from build123d import *

# Parameters (mm, degrees)
SKETCH_1_W      = 450
SKETCH_1_H      = 400
EXTRUDE_1_DEPTH = 50
SKETCH_2_W      = 50
SKETCH_2_H      = 50
EXTRUDE_2_DEPTH = 450
SKETCH_3_W      = 50
SKETCH_3_H      = 50
EXTRUDE_3_DEPTH = 450
SKETCH_4_W      = 50
SKETCH_4_H      = 50
EXTRUDE_4_DEPTH = 450
SKETCH_5_W      = 50
SKETCH_5_H      = 50
EXTRUDE_5_DEPTH = 450
SKETCH_6_W      = 400
SKETCH_6_H      = 80
EXTRUDE_6_DEPTH = 400
SKETCH_7_W      = 80
SKETCH_7_H      = 350
EXTRUDE_7_DEPTH = 250
SKETCH_8_W      = 80
SKETCH_8_H      = 350
EXTRUDE_8_DEPTH = 250


with BuildPart() as part:
    # 草图1 → 凸台-拉伸1 (new body)
    with BuildSketch(Plane.XY):
        Rectangle(SKETCH_1_W, SKETCH_1_H)
    extrude(amount=EXTRUDE_1_DEPTH)

    # 草图2 → 凸台-拉伸2 (add)
    with BuildSketch(Plane.XY):
        with Locations((-200, -175)):
            Rectangle(SKETCH_2_W, SKETCH_2_H)
    extrude(amount=EXTRUDE_2_DEPTH)

    # 草图3 → 凸台-拉伸3 (add)
    with BuildSketch(Plane.XY):
        with Locations((200, -175)):
            Rectangle(SKETCH_3_W, SKETCH_3_H)
    extrude(amount=EXTRUDE_3_DEPTH)

    # 草图4 → 凸台-拉伸4 (add)
    with BuildSketch(Plane.XY):
        with Locations((-200, 175)):
            Rectangle(SKETCH_4_W, SKETCH_4_H)
    extrude(amount=EXTRUDE_4_DEPTH)

    # 草图5 → 凸台-拉伸5 (add)
    with BuildSketch(Plane.XY):
        with Locations((200, 175)):
            Rectangle(SKETCH_5_W, SKETCH_5_H)
    extrude(amount=EXTRUDE_5_DEPTH)

    # 草图6 → 凸台-拉伸6 (add)
    with BuildSketch(Plane(origin=(0, 200, 0), x_dir=(1, 0, 0), z_dir=(0, 1, 0))):
        with Locations((0, -200)):
            Rectangle(SKETCH_6_W, SKETCH_6_H)
    extrude(amount=EXTRUDE_6_DEPTH)

    # 草图7 → 凸台-拉伸7 (add)
    with BuildSketch(Plane(origin=(0, 200, 0), x_dir=(1, 0, 0), z_dir=(0, 1, 0))):
        with Locations((-250, 0)):
            Rectangle(SKETCH_7_W, SKETCH_7_H)
    extrude(amount=EXTRUDE_7_DEPTH)

    # 草图8 → 凸台-拉伸8 (add)
    with BuildSketch(Plane(origin=(0, 200, 0), x_dir=(1, 0, 0), z_dir=(0, 1, 0))):
        with Locations((250, 0)):
            Rectangle(SKETCH_8_W, SKETCH_8_H)
    extrude(amount=EXTRUDE_8_DEPTH)


solid = part.part
Can you work these out from the model? Positions are in its coordinate system, mm. A direction names the side the tool comes from. Coordinates: 2 decimals unless noted, no trailing zeros. Order: outer loops, then holes, each group sorted by start corner. A loop starts at its lowest first (then second) coordinate and runs counter-clockwise, first axis right, second up. Notation, with made-up numbers: (-11, 21.5) - (30, 21.5) arc R27 cw to (30, 47.5) - close; hole circle Ø5 at (79.5, 38.25). An arc over 180 degrees is marked (long way). Answer as a JSON object with one key per item and string values. Group by question number.
Q1. I need wall thicknesses on line 1 (X direction, y = 431, z = -82.5); line 2 (Z direction, x = 185, y = 270.5); line 3 (Y direction, x = -205, z = 17). Which ranges of each line are inside material? Lowest first, please. Write a range as from..to.
Q2. Imagine slicing it at C-C (x = 31). Please give me the cut outline in (y, z), and give its area (3 significant figures).
Q3. Imagine slicing it at A-A (y = 297). Please give me the cut outline in (x, z), and give its area (3 significant figures).
Q4. On a 3-axis mill with a long thin cutter (end or side, diameter ignored), from which of +Z, -Z, +X, -X, +Y, -Y can I reach the whole of each face in a straight line? I mean faces 1 (the face through (-251, 323, 175)), 2 (the face through (200, -150, 247)), 3 (the face through (-200, 397, 201)), 4 (the face through (-18, -200, 41)). Say none if no direction works.
Q5. Imagine slicing it at D-D (z = 207.5). Please give me the cut outline in (x, y), and give its area (3 significant figures).
Q6. Imagine slicing it at B-B (z = -85). Please give me the cut outline in (x, y), and give its area (3 significant figures).
Q7. We'd pull the mould along X, two halves only. Please class faces 5 (the face through (200, 175, 450)), 6 (the face through (-175, 175, 247)), 7 (the face through (290, 323, 2)), 8 (the face through (175, 175, 247)): +X half, -X half, draft (parallel to the pull), parting line (faces both ways), or undercut.
Q8. Will these pins go through, and if not, where does the flat tip stop? P1, Ø25, axis at y = -177, z = 313.5, coming from the -X side; P2, Ø1, axis at x = 199.5, y = 177, coming from the -Z side; P3, Ø24, axis at y = 332, z = 201, coming from the -X side.
Determined:
{
 "1": {"line 1": "x = -290..-210, 210..290", "line 2": "z = 160..240", "line 3": "y = -200..200"},
 "2": {"outline": "(-200, 0) - (200, 0) - (200, 50) - (-200, 50) - close; (200, 160) - (600, 160) - (600, 240) - (200, 240) - close", "area": "52,000 mm2"},
 "3": {"outline": "(-290, -175) - (-210, -175) - (-210, 175) - (-290, 175) - close; (-200, 160) - (200, 160) - (200, 240) - (-200, 240) - close; (210, -175) - (290, -175) - (290, 175) - (210, 175) - close", "area": "88,000 mm2"},
 "4": {"face 1": "+Z, -X, +Y", "face 2": "+Z, +X, -X", "face 3": "+Z, -Z, +Y", "face 4": "+Z, -Z, +X, -X, -Y"},
 "5": {"outline": "(-225, -200) - (-175, -200) - (-175, -150) - (-225, -150) - close; (-225, 150) - (-175, 150) - (-175, 200) - (175, 200) - (175, 150) - (225, 150) - (225, 200) - (200, 200) - (200, 600) - (-200, 600) - (-200, 200) - (-225, 200) - close; (175, -200) - (225, -200) - (225, -150) - (175, -150) - close", "area": "170,000 mm2"},
 "6": {"outline": "(-290, 200) - (-210, 200) - (-210, 450) - (-290, 450) - close; (210, 200) - (290, 200) - (290, 450) - (210, 450) - close", "area": "40,000 mm2"},
 "7": {"face 5": "draft", "face 6": "undercut", "face 7": "+X half", "face 8": "undercut"},
 "8": {"P1": "stops at x = -225", "P2": "stops at z = 0", "P3": "stops at x = -200"}
}
